Geometry check sheet. Reference: the model listing, model coordinates, mm. Round coordinates to 2 decimals unless told otherwise and drop trailing zeros. Loops run counter-clockwise (first coordinate to the right, second up) from the corner with the lowest first, then second, coordinate; pieces in that order, holes last. Notation, with made-up numbers: M 33,79 L 71,79 A36 cw 71,115 Z; hole C -18,32 d9. An arc over 180 degrees is marked long. Use one line per item in the form item = value. Start each with the question number.
1. Material ranges on line 1 (Y direction, x = 48, z = 330); line 2 (X direction, y = 6.5, z = 277.5); line 3 (Z direction, x = 5.5, y = 30), recorded low to high.
2. Cross-section at C-C (x = 38.5). Record the boundary of the cut face in (y, z), then the cut area to 3 significant figures.
3. Go/stop test with flat-tipped pins: pin 1 (18.5 mm diameter, centred on y = 28.575, z = 330.2, fed in from -X); pin 2 (10 mm diameter, centred on x = 34.5, z = 473.5, fed in from +Y). Record where each tip stops, or that it passes through.
4. Cross-section at A-A (z = 330.2). Record the boundary of the cut face in (x, y), then the cut area to 3 significant figures.
5. Cross-section at B-B (z = 460.5). Record the boundary of the cut face in (x, y), then the cut area to 3 significant figures.
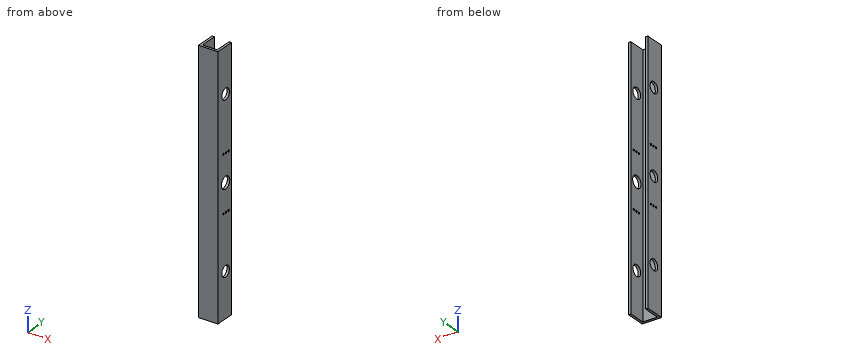
Autodesk Inventor part; units mm, degrees
ref_plane "YZ Plane" through (0, 0, 0) normal (1, 0, 0) x (0, 1, 0)
ref_plane "XZ Plane" through (0, 0, 0) normal (0, 1, 0) x (-1, 0, 0)
ref_plane "XY Plane" through (0, 0, 0) normal (0, 0, 1) x (1, 0, 0)
sketch "Sketch1" plane through (0, 0, 0) normal (0, 0, 1) x (1, 0, 0)
  line L0 (0, 0) -> (6.35, 0)
  line L1 (6.35, 0) -> (6.35, 50.8)
  line L2 (6.35, 50.8) -> (0, 50.8)
  line L3 (0, 50.8) -> (0, 0)
  line L4 (0, 0) -> (50.8, 0)
  line L5 (50.8, 0) -> (50.8, 6.35)
  line L6 (50.8, 6.35) -> (0, 6.35)
  line L7 (0, 6.35) -> (0, 0)
  line L8 (50.8, 0) -> (44.45, 0)
  line L9 (44.45, 0) -> (44.45, 50.8)
  line L10 (44.45, 50.8) -> (50.8, 50.8)
  line L11 (50.8, 50.8) -> (50.8, 0)
  dimension "d0" = 6.35
  dimension "d1" = 50.8
  dimension "d2" = 50.8
  dimension "d3" = 6.35
  dimension "d4" = 6.35
extrude "Extrusion1" add sketch "Sketch1" along normal blind 660.4
sketch "Sketch2" plane through (50.8, 0, 0) normal (1, 0, 0) x (0, 0, -1)
  line L0 (0, 0) -> (0, 6.35)
  line L1 (0, 0) -> (0, 50.8)
  line L2 (0, 6.35) -> (-660.4, 6.35)
  line L3 (0, 0) -> (-660.4, 0)
  line L4 (0, 6.35) -> (0, 50.8)
  line L5 (0, 28.575) -> (-115.189, 28.575)
  circle A0 centre (-115.189, 28.575) radius 14.2875
  line L6 (-660.4, 6.35) -> (-660.4, 50.8)
  line L7 (-660.4, 28.575) -> (-545.211, 28.575)
  circle A1 centre (-545.211, 28.575) radius 14.2875
  line L8 (0, 50.8) -> (-660.4, 50.8)
  line L9 (-330.2, 50.8) -> (-330.2, 28.575)
  circle A2 centre (-330.2, 28.575) radius 14.2875
  dimension "d7" = 6.35
  dimension "d8" = 115.189
  dimension "d9" = 28.575
  dimension "d10" = 115.189
  dimension "d11" = 28.575
extrude "Extrusion2" cut sketch "Sketch2" against normal blind 660.4 contours A0 | A2 | A1
sketch "Sketch3" plane through (50.8, 0, 0) normal (1, 0, 0) x (0, 0, -1)
  circle A0 centre (-330.2, 28.575) radius 14.2875
  circle A1 centre (-330.2, 28.575) radius 15.5575
  point P0 (0, 0)
  dimension "d14" = 31.115
extrude "Extrusion3" cut sketch "Sketch3" against normal blind 25.4
sketch "Sketch4" plane through (50.8, 0, 0) normal (1, 0, 0) x (0, 0, -1)
  circle A0 centre (-330.2, 28.575) radius 15.5575
  line L0 (-330.2, 28.575) -> (-330.2, 50.8)
  line L1 (0, 50.8) -> (-660.4, 50.8)
  line L2 (-330.2, 50.8) -> (-402.463, 50.8)
  line L3 (-402.463, 50.8) -> (-402.463, 39.6748)
  line L4 (-402.463, 39.6748) -> (-402.463, 30.1498)
  line L5 (-402.463, 30.1498) -> (-402.463, 20.6248)
  line L6 (-330.2, 50.8) -> (-257.937, 50.8)
  line L7 (-257.937, 50.8) -> (-257.937, 39.6748)
  line L8 (-257.937, 39.6748) -> (-257.937, 30.1498)
  line L9 (-257.937, 30.1498) -> (-257.937, 20.6248)
  circle A1 centre (-402.463, 39.6748) radius 2.54
  circle A2 centre (-402.463, 30.1498) radius 2.54
  circle A3 centre (-402.463, 20.6248) radius 2.54
  circle A4 centre (-257.937, 39.6748) radius 2.54
  circle A5 centre (-257.937, 30.1498) radius 2.54
  circle A6 centre (-257.937, 20.6248) radius 2.54
  point P0 (0, 0)
  dimension "d17" = 72.263
  dimension "d18" = 11.1252
  dimension "d19" = 9.525
  dimension "d20" = 9.525
  dimension "d21" = 72.263
  dimension "d22" = 5.08
extrude "Extrusion4" cut sketch "Sketch4" against normal blind 84.1375 contours A3 | A2 L5 L4 | L4 L5 A2 | A1 L4 L3 | L3 L4 A1 | A6 | A5 L9 L8 | L8 L9 A5 | A4 L8 L7 | L7 L8 A4
properties part number "U" material "Aluminum 6061"
Reported:
q1.line_1 = 0 to 13.02, 44.13 to 50.8
q1.line_2 = 0 to 6.35, 44.45 to 50.8
q1.line_3 = 0 to 100.97, 129.41 to 255.4, 260.47 to 315.98, 344.42 to 399.93, 405 to 530.99, 559.43 to 660.4
q2.outline = M 0,0 L 6.35,0 L 6.35,660.4 L 0,660.4 Z
q2.area = 4,190 mm²
q3.pin_1 = through
q3.pin_2 = 6.35
q4.outline = M 0,0 L 50.8,0 L 50.8,13.02 L 44.45,13.02 L 44.45,6.35 L 6.35,6.35 L 6.35,14.29 L 0,14.29 Z; M 0,42.86 L 6.35,42.86 L 6.35,50.8 L 0,50.8 Z; M 44.45,44.13 L 50.8,44.13 L 50.8,50.8 L 44.45,50.8 Z
q4.area = 508 mm²
q5.outline = M 0,0 L 50.8,0 L 50.8,50.8 L 44.45,50.8 L 44.45,6.35 L 6.35,6.35 L 6.35,50.8 L 0,50.8 Z
q5.area = 887 mm²
